The listing builds one solid part. Answer for the finished solid, in the listing's coordinates (mm). A direction names the side the tool comes from. Give positions to 0.01 mm unless a question says otherwise; leave off trailing zeros. Order: outer loops, then holes, each group sorted by start corner. A loop starts at its lowest first (then second) coordinate and runs counter-clockwise, first axis right, second up. Notation, with made-up numbers: (-21, 34.5) - (31, 34.5) arc R31 ccw to (31, 71.5) - close; hole circle Ø1 at (52.25, 35.25). An arc over 180 degrees is marked (long way). Use a Markdown table: item, result. Add a question column.
1) Straight lines are drawn through the part: line 1 (Y direction, x = -29, z = -15.75); line 2 (X direction, y = -40, z = -12.5) (3 decimals); line 3 (X direction, y = -3, z = -16) (3 decimals). For each, find the intervals that lie inside material, in ascending order.
2) Find section B-B, the plane z = -2. Determine the outline of the cut face in (x, y) (1 decimal), plus the area to 3 significant figures.
3) Flat-ended cylindrical pins translate along their axes: pin 1 (1 mm diameter, centred on x = 15.5, y = -10, fed in from +Z); pin 2 (5.5 mm diameter, centred on x = -1, y = 31, fed in from +Z); pin 3 (6 mm diameter, centred on x = -3, y = 13.5, fed in from +Z); pin 4 (4 mm diameter, centred on x = -28.75, y = 38.1, fed in from +Z). Find the tip coordinate at first contact, or state that the pin passes through.
4) For faces 5 (the face through (0, 32, -16.51)), 6 (the face through (0, 34.29, -18)), 7 (the face through (30.63, -36.37, -10.95)), determine the directions among +Z, -Z, +X, -X, +Y, -Y from which every point of the face is accessible in a straight line to the end or side of a thin tool.
5) Find section A-A, the plane y = 38.1. Determine the outline of the cut face in (x, z) (1 decimal), plus the area to 3 significant figures.
6) Find section D-D, the plane z = -10.5. Determine the outline of the cut face in (x, y) (1 decimal), plus the area to 3 significant figures.
7) Find section C-C, the plane x = 0. Determine the outline of the cut face in (y, z), plus the area to 3 significant figures.
8) The mould has two halves that part along X. Classify faces 1 (the face through (-28.199, 35.608, -10.946)), 2 (the face through (0, 29.21, -18)), 3 (the face through (-1, 1, -21.59)), 4 (the face through (37.465, -1, -11)): released by +X, released by -X, zero draft, split by the parting line, or undercut.
from build123d import *

# Parameters (mm, degrees)
SKETCH1_W                   = 74.93
SKETCH1_H                   = 101.6
BOSS_EXTRUDE2_DEPTH         = 21.59
CUT_EXTRUDE2_DEPTH          = 111.418813275
CUT_EXTRUDE2_DEPTH_BACK     = 111.418813275
SKETCH4_W                   = 7.62
SKETCH4_H                   = 5.08
BOSS_EXTRUDE3_DEPTH         = 2.54
TAP_DRILL_FOR_1_4_20_TAP1_D = 5.1054


with BuildPart() as part:
    # Sketch1 → Boss-Extrude2 (new body)
    with BuildSketch(Plane.XY):
        Rectangle(SKETCH1_W, SKETCH1_H)
    extrude(amount=-BOSS_EXTRUDE2_DEPTH)

    # Sketch2 → Cut-Extrude2 (cut, two sides: drawn at the far end of the back side and taken through both)
    with BuildSketch(Plane(origin=(0, 50.8, 0), x_dir=(1, 0, 0), z_dir=(0, 1, 0)).offset(-CUT_EXTRUDE2_DEPTH_BACK)):
        with BuildLine():
            Line((-18.542, -130.048526005), (-18.542, 0))
            ThreePointArc((-18.542, 0), (0, 18.542), (18.542, 0))
            Line((18.542, 0), (18.542, -130.048526005))
            Line((18.542, -130.048526005), (18.542, -390.145578015))
            Line((18.542, -390.145578015), (-18.542, -390.145578015))
            Line((-18.542, -390.145578015), (-18.542, -130.048526005))
        make_face()
    extrude(amount=CUT_EXTRUDE2_DEPTH + CUT_EXTRUDE2_DEPTH_BACK, mode=Mode.SUBTRACT)

    # Sketch4 → Boss-Extrude3 (add, symmetric)
    with BuildSketch(Plane(origin=(0, 31.75, 0), x_dir=(1, 0, 0), z_dir=(0, 1, 0))):
        with Locations((0, 19.05)):
            Rectangle(SKETCH4_W, SKETCH4_H)
    extrude(amount=BOSS_EXTRUDE3_DEPTH, both=True)

    # Tap Drill for 1/4-20 Tap1 (through all)
    with Locations(Plane.XY):
        with Locations((-28.7528, 38.1), (28.7528, 38.1), (-28.7528, -38.1), (28.7528, -38.1)):
            Hole(TAP_DRILL_FOR_1_4_20_TAP1_D / 2)


solid = part.part
The answers:
| question | item | result |
|---|---|---|
| 1 | line 1 | -50.8 to -40.64, -35.56 to 35.56, 40.64 to 50.8 |
| 1 | line 2 | -37.465 to -30.458, -27.048 to -13.695, 13.695 to 27.048, 30.458 to 37.465 |
| 1 | line 3 | -37.465 to -9.37, 9.37 to 37.465 |
| 2 | outline | (-37.5, -50.8) - (-18.4, -50.8) - (-18.4, 50.8) - (-37.5, 50.8) - close; (18.4, -50.8) - (37.5, -50.8) - (37.5, 50.8) - (18.4, 50.8) - close; hole circle Ø5.1 at (-28.8, -38.1); hole circle Ø5.1 at (-28.8, 38.1); hole circle Ø5.1 at (28.8, -38.1); hole circle Ø5.1 at (28.8, 38.1) |
| 2 | area | 3,790 mm2 |
| 3 | pin 1 | z = -9.37 |
| 3 | pin 2 | z = -16.51 |
| 3 | pin 3 | z = -17.54 |
| 3 | pin 4 | through |
| 4 | face 5 | +Z, +Y, -Y |
| 4 | face 6 | +Z, +Y |
| 4 | face 7 | +Z, -Z |
| 5 | outline | (-37.5, -21.6) - (-31.3, -21.6) - (-31.3, 0) - (-37.5, 0) - close; (-26.2, -21.6) - (26.2, -21.6) - (26.2, 0) - (18.5, 0) arc R18.5 cw to (-18.5, 0) - (-26.2, 0) - close; (31.3, -21.6) - (37.5, -21.6) - (37.5, 0) - (31.3, 0) - close |
| 5 | area | 857 mm2 |
| 6 | outline | (-37.5, -50.8) - (-15.3, -50.8) - (-15.3, 50.8) - (-37.5, 50.8) - close; (15.3, -50.8) - (37.5, -50.8) - (37.5, 50.8) - (15.3, 50.8) - close; hole circle Ø5.1 at (-28.8, -38.1); hole circle Ø5.1 at (-28.8, 38.1); hole circle Ø5.1 at (28.8, -38.1); hole circle Ø5.1 at (28.8, 38.1) |
| 6 | area | 4,430 mm2 |
| 7 | outline | (-50.8, -21.59) - (50.8, -21.59) - (50.8, -18.54) - (34.29, -18.54) - (34.29, -16.51) - (29.21, -16.51) - (29.21, -18.54) - (-50.8, -18.54) - close |
| 7 | area | 320 mm2 |
| 8 | face 1 | undercut |
| 8 | face 2 | undercut |
| 8 | face 3 | zero draft |
| 8 | face 4 | released by +X |
